from build123d import *

# Parameters (mm, degrees)
SKETCH_R  = 1.5625
PAD_DEPTH = 12
FILLET_R  = 3


with BuildPart() as part:
    # Sketch → Pad (new body)
    with BuildSketch(Plane.XY):
        Polygon((400, -50), (0, -50), (0, 0), (-160, 0), (-160, 320), (400, 320), align=None)
        with Locations((85, 15)):
            Circle(SKETCH_R, mode=Mode.SUBTRACT)
        with Locations((105, 15)):
            Circle(SKETCH_R, mode=Mode.SUBTRACT)
        with Locations((75, 25)):
            Circle(SKETCH_R, mode=Mode.SUBTRACT)
        with Locations((95, 25)):
            Circle(SKETCH_R, mode=Mode.SUBTRACT)
        with Locations((155, 15)):
            Circle(SKETCH_R, mode=Mode.SUBTRACT)
        with Locations((135, 15)):
            Circle(SKETCH_R, mode=Mode.SUBTRACT)
        with Locations((145, 25)):
            Circle(SKETCH_R, mode=Mode.SUBTRACT)
        with Locations((165, 25)):
            Circle(SKETCH_R, mode=Mode.SUBTRACT)
        with Locations((85, 185)):
            Circle(SKETCH_R, mode=Mode.SUBTRACT)
        with Locations((105, 185)):
            Circle(SKETCH_R, mode=Mode.SUBTRACT)
        with Locations((75, 175)):
            Circle(SKETCH_R, mode=Mode.SUBTRACT)
        with Locations((95, 175)):
            Circle(SKETCH_R, mode=Mode.SUBTRACT)
        with Locations((155, 185)):
            Circle(SKETCH_R, mode=Mode.SUBTRACT)
        with Locations((135, 185)):
            Circle(SKETCH_R, mode=Mode.SUBTRACT)
        with Locations((145, 175)):
            Circle(SKETCH_R, mode=Mode.SUBTRACT)
        with Locations((165, 175)):
            Circle(SKETCH_R, mode=Mode.SUBTRACT)
        with Locations((225, 185)):
            Circle(SKETCH_R, mode=Mode.SUBTRACT)
        with Locations((205, 185)):
            Circle(SKETCH_R, mode=Mode.SUBTRACT)
        with Locations((235, 175)):
            Circle(SKETCH_R, mode=Mode.SUBTRACT)
        with Locations((215, 175)):
            Circle(SKETCH_R, mode=Mode.SUBTRACT)
        with Locations((175, 185)):
            Circle(SKETCH_R, mode=Mode.SUBTRACT)
        with Locations((235, 25)):
            Circle(SKETCH_R, mode=Mode.SUBTRACT)
        with Locations((215, 25)):
            Circle(SKETCH_R, mode=Mode.SUBTRACT)
        with Locations((205, 15)):
            Circle(SKETCH_R, mode=Mode.SUBTRACT)
        with Locations((225, 15)):
            Circle(SKETCH_R, mode=Mode.SUBTRACT)
        with Locations((245, 15)):
            Circle(SKETCH_R, mode=Mode.SUBTRACT)
        with Locations((255, 25)):
            Circle(SKETCH_R, mode=Mode.SUBTRACT)
        with Locations((245, 185)):
            Circle(SKETCH_R, mode=Mode.SUBTRACT)
        with Locations((255, 175)):
            Circle(SKETCH_R, mode=Mode.SUBTRACT)
    extrude(amount=PAD_DEPTH)

    # Fillet
    fillet_edges = [part.edges().sort_by_distance(p)[0] for p in [
        (400, -50, 6),
        (0, -50, 6),
        (0, 0, 6),
        (-160, 0, 6),
    ]]
    fillet(fillet_edges, radius=FILLET_R)


solid = part.part
Model file for the job. Use its own axes, mm. A direction names the side the tool comes from. Coordinates: 2 decimals unless noted, no trailing zeros. Write each loop counter-clockwise with the first axis right and the second up, starting at its lowest first coordinate (ties: lowest second). Pieces come first, ordered by that corner, then holes. Notation, with made-up numbers: (-5.5, 87) - (36.5, 87) arc R11 cw to (36.5, 100) - close; hole circle Ø11 at (43, 21.5). An arc over 180 degrees is marked (long way). Write each question's results on one line, items separated by ' | '. Start each with the question number.
1) Cut at A-A (z = 2.25). Count the separate pieces of the cut face and the enclosed holes in it, then the cut area to 3 significant figures.
2) Flat gauge pins, fed straight in: P1, Ø3, axis at x = 255, y = 25, coming from the -Z side; P2, Ø5, axis at x = -33, z = 5.5, coming from the -Y side. Where does each tip first touch, or does it go through?
3) Probe line 1 along Y through (x, z) = (215, 4.75); line 2 along Y through (x, z) = (105, 4.25); line 3 along Y through (x, z) = (175, 7.5). List the from-to ranges inside material, lowest first. Write a range as from..to.
4) Cut at B-B (y = -11). Write the cut outline in (x, z).
5) 3-axis set-ups, long thin cutter, end or side, ignore diameter. For faces 1 (the face through (0, -25, 6)), 2 (the face through (124, 138, 0)): which of +Z, -Z, +X, -X, +Y, -Y reach the whole face in a straight line?
Returned:
1) separate pieces: 1 | enclosed holes: 29 | area: 199,000 mm^2
2) P1: through | P2: y = 0
3) line 1: -50..23.44, 26.56..173.44, 176.56..320 | line 2: -50..13.44, 16.56..183.44, 186.56..320 | line 3: -50..183.44, 186.56..320
4) outline: (0, 0) - (400, 0) - (400, 12) - (0, 12) - close
5) face 1: +Z, -Z, -X, -Y | face 2: -Z, +X, -X, +Y, -Y
